```python
from build123d import *

# Parameters (mm, degrees)
SKETCH1_W            = 186
SKETCH1_H            = 166
BOSS_EXTRUDE6_DEPTH  = 3
SKETCH9_W            = 183
SKETCH9_H            = 3
BOSS_EXTRUDE7_DEPTH  = 105
SKETCH8_W            = 3
SKETCH8_H            = 163
BOSS_EXTRUDE8_DEPTH  = 105
SKETCH7_W            = 186
SKETCH7_H            = 3
BOSS_EXTRUDE9_DEPTH  = 105
SKETCH11_W           = 3
SKETCH11_H           = 160
BOSS_EXTRUDE10_DEPTH = 105
SKETCH12_W           = 180
SKETCH12_H           = 3
BOSS_EXTRUDE11_DEPTH = 20
SKETCH13_W           = 45
SKETCH13_H           = 8
CUT_EXTRUDE5_DEPTH   = 3
SKETCH20_W           = 3
SKETCH20_H           = 2
BOSS_EXTRUDE12_DEPTH = 50
SKETCH18_W           = 20
SKETCH18_H           = 20
CUT_EXTRUDE6_DEPTH   = 3
SKETCH22_W           = 3
SKETCH22_H           = 30
BOSS_EXTRUDE13_DEPTH = 6.5
SKETCH23_W           = 3
SKETCH23_H           = 30
BOSS_EXTRUDE15_DEPTH = 20
SKETCH24_R           = 2.5
CUT_EXTRUDE8_DEPTH   = 10


with BuildPart() as part:
    # Sketch1 → Boss-Extrude6 (new body)
    with BuildSketch(Plane(origin=(0, 0, 0), x_dir=(1, 0, 0), z_dir=(0, 1, 0))):
        with Locations((3.75, -30.125)):
            Rectangle(SKETCH1_W, SKETCH1_H)
    extrude(amount=BOSS_EXTRUDE6_DEPTH)

    # Sketch9 → Boss-Extrude7 (add)
    with BuildSketch(Plane(origin=(0, 3, 0), x_dir=(1, 0, 0), z_dir=(0, 1, 0))):
        with Locations((2.25, -111.625)):
            Rectangle(SKETCH9_W, SKETCH9_H)
    extrude(amount=BOSS_EXTRUDE7_DEPTH)

    # Sketch8 → Boss-Extrude8 (add)
    with BuildSketch(Plane(origin=(0, 3, 0), x_dir=(1, 0, 0), z_dir=(0, 1, 0))):
        with Locations((95.25, -31.625)):
            Rectangle(SKETCH8_W, SKETCH8_H)
    extrude(amount=BOSS_EXTRUDE8_DEPTH)

    # Sketch7 → Boss-Extrude9 (add)
    with BuildSketch(Plane(origin=(0, 3, 0), x_dir=(1, 0, 0), z_dir=(0, 1, 0))):
        with Locations((3.75, 51.375)):
            Rectangle(SKETCH7_W, SKETCH7_H)
    extrude(amount=BOSS_EXTRUDE9_DEPTH)

    # Sketch11 → Boss-Extrude10 (add)
    with BuildSketch(Plane(origin=(0, 3, 0), x_dir=(1, 0, 0), z_dir=(0, 1, 0))):
        with Locations((-87.75, -30.125)):
            Rectangle(SKETCH11_W, SKETCH11_H)
    extrude(amount=BOSS_EXTRUDE10_DEPTH)

    # Sketch12 → Boss-Extrude11 (add)
    with BuildSketch(Plane(origin=(0, 3, 0), x_dir=(1, 0, 0), z_dir=(0, 1, 0))):
        with Locations((3.75, -52.625)):
            Rectangle(SKETCH12_W, SKETCH12_H)
    extrude(amount=BOSS_EXTRUDE11_DEPTH)

    # Sketch13 → Cut-Extrude5 (cut)
    with BuildSketch(Plane(origin=(-86.25, 0, 0), x_dir=(0, 0, -1), z_dir=(1, 0, 0))):
        with Locations((25.375, 7)):
            Rectangle(SKETCH13_W, SKETCH13_H)
    extrude(amount=-CUT_EXTRUDE5_DEPTH, mode=Mode.SUBTRACT)

    # Sketch20 → Boss-Extrude12 (add)
    with BuildSketch(Plane(origin=(0, 3, 0), x_dir=(1, 0, 0), z_dir=(0, 1, 0))):
        with Locations((-81.25, 48.875)):
            Rectangle(SKETCH20_W, SKETCH20_H)
    extrude(amount=BOSS_EXTRUDE12_DEPTH)

    # Sketch18 → Cut-Extrude6 (cut)
    with BuildSketch(Plane.ZY.offset(89.25)):
        with Locations((7.125, 13)):
            Rectangle(SKETCH18_W, SKETCH18_H)
    extrude(amount=-CUT_EXTRUDE6_DEPTH, mode=Mode.SUBTRACT)

    # Sketch22 → Boss-Extrude13 (add)
    with BuildSketch(Plane(origin=(-86.25, 0, 0), x_dir=(0, 0, -1), z_dir=(1, 0, 0))):
        with Locations((1.375, 38)):
            Rectangle(SKETCH22_W, SKETCH22_H)
    extrude(amount=BOSS_EXTRUDE13_DEPTH)

    # Sketch23 → Boss-Extrude15 (add)
    with BuildSketch(Plane(origin=(0, 0, -2.875), x_dir=(-1, 0, 0), z_dir=(0, 0, -1))):
        with Locations((81.25, 38)):
            Rectangle(SKETCH23_W, SKETCH23_H)
    extrude(amount=BOSS_EXTRUDE15_DEPTH)

    # Sketch24 → Cut-Extrude8 (cut)
    with BuildSketch(Plane.XY.offset(-49.875)):
        with Locations((-57.365874662, 67.44295955)):
            Circle(SKETCH24_R)
    extrude(amount=-CUT_EXTRUDE8_DEPTH, mode=Mode.SUBTRACT)


solid = part.part
```
Geometry check sheet. Reference: the model listing, model coordinates, mm. A direction names the side the tool comes from. Round coordinates to 2 decimals unless told otherwise and drop trailing zeros. Order: outer loops, then holes, each group sorted by start corner. A loop starts at its lowest first (then second) coordinate and runs counter-clockwise, first axis right, second up. Notation, with made-up numbers: (-19, 15) - (17, 15) arc R21 cw to (17, 50) - close; hole circle Ø1 at (-25.5, -19). An arc over 180 degrees is marked (long way). Use a Markdown table: item, result. Add a question column.
(1) Sectioned sample at A-A, the plane z = -35.5. Enter the section's corners in (x, y), and give its area (3 significant figures).
(2) Sectioned sample at D-D, the plane z = 97.5. Enter the section's corners in (x, y).
(3) Depth check by flat-ended pin: pin 1 (17 mm diameter, centred on x = 31.5, z = 94, fed in from +Y); pin 2 (2 mm diameter, centred on x = -82, z = -11.5, fed in from +Y); pin 3 (5 mm diameter, centred on x = 48.5, z = -18, fed in from -Y). Enter the tip coordinate at first touch or a pass-through.
(4) Tool access check on faces 1 (the flat face through (2, 13, 54.125)), 2 (the cylindrical face through (-57.9, 65, -51.4)), 3 (the flat face through (2, 53, 113.125)). Record the directions out of +Z, -Z, +X, -X, +Y, -Y that give a thin tool (end or side, any length) a straight path to the whole face; none if there is none.
(5) Release check for a two-part mould opening along X. For faces 4 (the flat face through (-86.25, 55, 31)), 5 (the flat face through (-89.25, 53, 31)), 6 (the flat face through (2, 55, -49.875)), 7 (the flat face through (96.75, 53, 31)) record: pulls with the +X half, pulls with the -X half, needs draft (parallel to the pull), parting line crosses it, or undercut.
(6) Material ranges on line 1 along Z through (x, y) = (54, 14.5) (3 decimals); line 2 along Z through (x, y) = (75.5, 83) (3 decimals); line 3 along X through (y, z) = (100, 91), recorded low to high. Write a range as [from, to].
(7) Sectioned sample at C-C, the plane x = 13. Enter the section's corners in (y, z) (3 decimals).
(8) Sectioned sample at B-B, the plane y = 30.5. Enter the section's corners in (x, z) (3 decimals), and give its area (3 significant figures).
Answers below:
| question | item | result |
|---|---|---|
| 1 | outline | (-89.25, 0) - (96.75, 0) - (96.75, 108) - (93.75, 108) - (93.75, 3) - (-89.25, 3) - close; (-89.25, 11) - (-86.25, 11) - (-86.25, 108) - (-89.25, 108) - close |
| 1 | area | 1,160 mm² |
| 2 | outline | (-89.25, 0) - (96.75, 0) - (96.75, 108) - (93.75, 108) - (93.75, 3) - (-86.25, 3) - (-86.25, 108) - (-89.25, 108) - close |
| 3 | pin 1 | y = 3 |
| 3 | pin 2 | y = 53 |
| 3 | pin 3 | y = 0 |
| 4 | face 1 | +Y |
| 4 | face 2 | -Z |
| 4 | face 3 | +Z, +X, -X, +Y, -Y |
| 5 | face 4 | undercut |
| 5 | face 5 | pulls with the -X half |
| 5 | face 6 | undercut |
| 5 | face 7 | pulls with the +X half |
| 6 | line 1 | [-52.875, -49.875], [51.125, 54.125], [110.125, 113.125] |
| 6 | line 2 | [-52.875, -49.875], [110.125, 113.125] |
| 6 | line 3 | [-89.25, -86.25], [93.75, 96.75] |
| 7 | outline | (0, -52.875) - (108, -52.875) - (108, -49.875) - (3, -49.875) - (3, 51.125) - (23, 51.125) - (23, 54.125) - (3, 54.125) - (3, 110.125) - (108, 110.125) - (108, 113.125) - (0, 113.125) - close |
| 8 | outline | (-89.25, -52.875) - (96.75, -52.875) - (96.75, 113.125) - (-89.25, 113.125) - close; hole (-86.25, -49.875) - (-82.75, -49.875) - (-82.75, -47.875) - (-79.75, -47.875) - (-79.75, -49.875) - (93.75, -49.875) - (93.75, 110.125) - (-86.25, 110.125) - (-86.25, 0.125) - (-79.75, 0.125) - (-79.75, -22.875) - (-82.75, -22.875) - (-82.75, -2.875) - (-86.25, -2.875) - close |
| 8 | area | 2,160 mm² |
